from build123d import *

# Parameters (mm, degrees)
SKETCH1_R           = 3.96875
SKETCH1_R_2         = 15.08125
SKETCH1_R_3         = 2
BOSS_EXTRUDE1_DEPTH = 6.35


with BuildPart() as part:
    # Sketch1 → Boss-Extrude1 (new body)
    with BuildSketch(Plane(origin=(0, 0, 0), x_dir=(1, 0, 0), z_dir=(0, 1, 0))):
        with BuildLine():
            Line((25.4, -39.926769414), (25.4, -173.650783549))
            ThreePointArc((25.4, -173.650783549), (25.170228885, -174.953880295), (24.508629328, -176.099804342))
            Line((24.508629328, -176.099804342), (-20.914247114, -230.232680529))
            ThreePointArc((-20.914247114, -230.232680529), (-23.728731164, -230.986819257), (-25.4, -228.6))
            Line((-25.4, -228.6), (-25.4, -39.926769414))
            ThreePointArc((-25.4, -39.926769414), (-25.169027772, -38.620377357), (-24.504115377, -37.472379149))
            add(Edge.make_bspline(
                [(-24.504115377, -37.472379149), (-15.341464403, -26.593497135), (-9.143369894, -14.104472305), (-6.985, 0)],
                knots=[0.031078099, 0.031078099, 0.031078099, 0.031078099, 1, 1, 1, 1], degree=3))
            ThreePointArc((-6.985, 0), (0, 6.985), (6.985, 0))
            add(Edge.make_bspline(
                [(24.504115377, -37.472379149), (15.363034866, -26.619107902), (9.178211427, -14.199965817), (6.985, 0)],
                knots=[0.031766068, 0.031766068, 0.031766068, 0.031766068, 1, 1, 1, 1], degree=3))
            ThreePointArc((24.504115377, -37.472379149), (25.169027772, -38.620377357), (25.4, -39.926769414))
        make_face()
        with Locations(Location((0, 0, 0), (0, 0, 270))):
            Circle(SKETCH1_R, mode=Mode.SUBTRACT)
        with Locations(Location((0, -138.43, 0), (0, 0, 270))):
            Circle(SKETCH1_R_2, mode=Mode.SUBTRACT)
        with Locations(Location((-20.32, -222.878592645, 0), (0, 0, 270))):
            Circle(SKETCH1_R_3, mode=Mode.SUBTRACT)
        with Locations(Location((-20.32, -216.528592645, 0), (0, 0, 270))):
            Circle(SKETCH1_R_3, mode=Mode.SUBTRACT)
        with Locations(Location((-20.32, -210.178592645, 0), (0, 0, 270))):
            Circle(SKETCH1_R_3, mode=Mode.SUBTRACT)
        with Locations(Location((-20.32, -203.828592645, 0), (0, 0, 270))):
            Circle(SKETCH1_R_3, mode=Mode.SUBTRACT)
        with Locations(Location((21.59, -173.650783549, 0), (0, 0, 270))):
            Circle(SKETCH1_R_3, mode=Mode.SUBTRACT)
        with Locations(Location((8.19455983, -25.4, 0), (0, 0, 270))):
            Circle(SKETCH1_R_3, mode=Mode.SUBTRACT)
        with BuildLine():
            Line((5.605496622, -176.452263434), (-13.166879596, -150.15491695))
            ThreePointArc((-13.166879596, -150.15491695), (-13.808086261, -149.684948511), (-14.603073846, -149.688274478))
            Line((-14.603073846, -149.688274478), (-18.395861473, -150.955793975))
            ThreePointArc((-18.395861473, -150.955793975), (-19.045805463, -151.449552817), (-19.26101006, -152.2368977))
            Line((-19.26101006, -152.2368977), (-16.771936742, -193.436924326))
            ThreePointArc((-16.771936742, -193.436924326), (-12.825939472, -198.936057494), (-6.161826947, -197.752434107))
            Line((-6.161826947, -197.752434107), (4.350250475, -188.195205906))
            ThreePointArc((4.350250475, -188.195205906), (7.209558699, -182.562287673), (5.605496622, -176.452263434))
        make_face(mode=Mode.SUBTRACT)
        with BuildLine():
            Line((-12.7, -120.970386602), (-5.976567434, -102.241338504))
            ThreePointArc((-5.976567434, -102.241338504), (0, -98.036831852), (5.976567434, -102.241338504))
            Line((5.976567434, -102.241338504), (12.7, -120.970386602))
            ThreePointArc((12.7, -120.970386602), (0, -116.84), (-12.7, -120.970386602))
        make_face(mode=Mode.SUBTRACT)
    extrude(amount=-BOSS_EXTRUDE1_DEPTH)


solid = part.part
The model under review builds one solid part; all positions refer to its coordinate system, in mm. A direction names the side the tool comes from. Give positions to 0.01 mm unless a question says otherwise; leave off trailing zeros. Loops run counter-clockwise (first coordinate to the right, second up) from the corner with the lowest first, then second, coordinate; pieces in that order, holes last. Notation, with made-up numbers: (65, -17.5) -> (113, -17.5) arc R24 ccw to (113, 20.5) -> close; hole circle Ø6 at (53.25, -7). An arc over 180 degrees is marked (long way). Answer as a JSON object with one key per item and string values. Group by question number.
Q1. Take a section at B-B (x = 0). Write out the cut boundary in (y, z) (3 decimals), plus the area to 3 significant figures.
Q2. Wall thickness on line 1 along Z through (x, y) = (-22, -1); line 2 along X through (y, z) = (-2.75, 138.43); line 3 along Z through (x, y) = (-20, -5.25): over which ranges is each line inside the solid? List them lowest first.
Q3. Draft analysis for pull direction X (two halves, no side actions). For faces 1 (the cylindrical face through (0.663, -3.131, 123.363)), 2 (the flat face through (0, -6.35, 84)), 3 (the cylindrical face through (-0.154, -3.131, -6.983)), state which applies: pulls with the +X half, pulls with the -X half, needs draft (parallel to the pull), parting line crosses it, or undercut.
Q4. Take a section at C-C (y = -2.5). State how many separate pieces and enclosed holes the cut face has, plus the area to 3 significant figures.
Q5. Take a section at A-A (z = 138.43). Write out the cut boundary in (x, y).
Q6. Tool access review of faces 4 (the cylindrical face through (-0.109, -3.131, 98.038)), 5 (the flat face through (-25.4, -3, 136)): name each direction out of +Z, -Z, +X, -X, +Y, -Y from which nothing blocks a thin tool from reaching the whole face with its end or side.
Answer below:
{
 "1": {"outline": "(-6.35, -6.985) -> (0, -6.985) -> (0, -3.969) -> (-6.35, -3.969) -> close; (-6.35, 3.969) -> (0, 3.969) -> (0, 98.037) -> (-6.35, 98.037) -> close; (-6.35, 116.84) -> (0, 116.84) -> (0, 123.349) -> (-6.35, 123.349) -> close; (-6.35, 153.511) -> (0, 153.511) -> (0, 168.6) -> (-6.35, 168.6) -> close; (-6.35, 192.15) -> (0, 192.15) -> (0, 205.308) -> (-6.35, 205.308) -> close", "area": "837 mm2"},
 "2": {"line 1": "z = 34.36 to 202.74, 204.91 to 209.09, 211.26 to 215.44, 217.61 to 221.79, 223.96 to 230.99", "line 2": "x = -25.4 to -15.08, 15.08 to 25.4", "line 3": "z = 31.65 to 201.85, 205.8 to 208.2, 212.15 to 214.55, 218.5 to 220.9, 224.85 to 229.14"},
 "3": {"face 1": "undercut", "face 2": "needs draft", "face 3": "parting line crosses it"},
 "4": {"separate pieces": "1", "enclosed holes": "10", "area": "7,630 mm2"},
 "5": {"outline": "(-25.4, -6.35) -> (-15.08, -6.35) -> (-15.08, 0) -> (-25.4, 0) -> close; (15.08, -6.35) -> (25.4, -6.35) -> (25.4, 0) -> (15.08, 0) -> close"},
 "6": {"face 4": "+Y, -Y", "face 5": "+Z, -Z, -X, +Y, -Y"}
}
